Could you check a few things on this model? Use its own coordinates, in mm. A direction names the side the tool comes from. Coordinates: 2 decimals unless noted, no trailing zeros. Order: outer loops, then holes, each group sorted by start corner. A loop starts at its lowest first (then second) coordinate and runs counter-clockwise, first axis right, second up. Notation, with made-up numbers: M 10.25,7 L 41.25,7 A21 cw 41.25,43 Z; hole C 38,30 d11. An arc over 180 degrees is marked long. Put each result on its own line as item: value. Start each with the question number.
```python
from build123d import *

# Parameters (mm, degrees)
EXTRUDE_3_DEPTH     = 13
SKETCH_5_R          = 2.1
CUT_EXTRUDE_2_DEPTH = 48.895720059
SKETCH_6_W          = 7.2
SKETCH_6_H          = 35
EXTRUDE_4_DEPTH     = 20
SKETCH_7_R          = 2.1
CUT_EXTRUDE_3_DEPTH = 20
SKETCH_8_W          = 22.8
SKETCH_8_H          = 3.5
EXTRUDE_5_DEPTH     = 10
SKETCH_9_R          = 6.65
CUT_EXTRUDE_4_DEPTH = 4.2
CUT_EXTRUDE_5_DEPTH = 10
CUT_EXTRUDE_6_DEPTH = 10
SKETCH_14_R         = 6.85
SKETCH_14_R_2       = 5.65
EXTRUDE_7_DEPTH     = 3


with BuildPart() as part:
    # 草图4 → 凸台-拉伸3 (new body)
    with BuildSketch(Plane.XY):
        Polygon((15, 0), (-15, 0), (-15, 35), (-7.8, 35), (-7.8, 3.5), (7.8, 3.5), (7.8, 35), (15, 35), align=None)
    extrude(amount=EXTRUDE_3_DEPTH)

    # 草图5 → 切除-拉伸2 (cut, through all)
    with BuildSketch(Plane(origin=(15, 0, 0), x_dir=(0, 0, -1), z_dir=(1, 0, 0))):
        with Locations(Location((-6.5, 30, 0), (0, 0, 90))):
            Circle(SKETCH_5_R)
    extrude(amount=-CUT_EXTRUDE_2_DEPTH, mode=Mode.SUBTRACT)

    # 草图6 → 凸台-拉伸4 (add)
    with BuildSketch(Plane.XY.offset(13)):
        with Locations((-11.4, 17.5)):
            Rectangle(SKETCH_6_W, SKETCH_6_H)
    extrude(amount=EXTRUDE_4_DEPTH)

    # 草图7 → 切除-拉伸3 (cut)
    with BuildSketch(Plane.ZY.offset(15)):
        with Locations(Location((23.849351573, 12, 0), (0, 0, 270))):
            Circle(SKETCH_7_R)
    extrude(amount=-CUT_EXTRUDE_3_DEPTH, mode=Mode.SUBTRACT)

    # 草图8 → 凸台-拉伸5 (add)
    with BuildSketch(Plane.XY.offset(13)):
        with Locations((3.6, 1.75)):
            Rectangle(SKETCH_8_W, SKETCH_8_H)
    extrude(amount=EXTRUDE_5_DEPTH)

    # 草图9 → 切除-拉伸4 (cut)
    with BuildSketch(Plane(origin=(-7.8, 0, 0), x_dir=(0, 0, -1), z_dir=(1, 0, 0))):
        with Locations(Location((-23.849351573, 12, 0), (0, 0, 90))):
            Circle(SKETCH_9_R)
    extrude(amount=-CUT_EXTRUDE_4_DEPTH, mode=Mode.SUBTRACT)

    # 草图10 → 切除-拉伸5 (cut)
    with BuildSketch(Plane.ZY.offset(15)):
        Polygon((12.890771142, 35), (31.03620252, 14.67169088), (31.03620252, 9.814342957), (24.670130024, 0), (33, 0), (33, 10.134215088), (33, 35), align=None)
        Polygon((0, 35), (0, 31.107929111), (4.419316467, 35), align=None)
    extrude(amount=-CUT_EXTRUDE_5_DEPTH, mode=Mode.SUBTRACT)

    # 草图11 → 切除-拉伸6 (cut)
    with BuildSketch(Plane(origin=(15, 0, 0), x_dir=(0, 0, -1), z_dir=(1, 0, 0))):
        Polygon((-3.336766509, 35), (0, 31.348169844), (0, 35), align=None)
        Polygon((-10.303751585, 35), (-13, 35), (-13, 31.657050955), align=None)
    extrude(amount=-CUT_EXTRUDE_6_DEPTH, mode=Mode.SUBTRACT)

    # 草图14 → 凸台-拉伸7 (add)
    with BuildSketch(Plane.ZY.offset(15)):
        with Locations(Location((23.849351573, 12, 0), (0, 0, 180))):
            Circle(SKETCH_14_R)
        with Locations((23.849351573, 12)):
            Circle(SKETCH_14_R_2, mode=Mode.SUBTRACT)
    extrude(amount=EXTRUDE_7_DEPTH)


solid = part.part
```
Item 1: If we section it at B-B on x = 8.5: Write out the boundary of the cut face in (y, z), then the cut area to 3 significant figures.
Item 2: If we section it at A-A on y = 12: Write out the boundary of the cut face in (x, z), then the cut area to 3 significant figures.
Item 3: If we section it at D-D on y = 30: Write out the boundary of the cut face in (x, z).
Item 4: If we mould it in two halves opening along Z, with no side actions, what happens to faces 1 (the flat face through (0, 0, 12)), 2 (the flat face through (10, 16, 0)), 3 (the flat face through (-12, 10, 25))? For each: released by +Z, released by -Z, zero draft, split by the parting line, or undercut.
Item 5: I need wall thicknesses on probe 1 along X at (y, z) = (5, 2); probe 2 along X at (y, z) = (24, 17); probe 3 along Z at (x, y) = (12, 23). Which ranges of each line are inside material? Lowest first, please.
Item 6: For pin 1 Ø2 at (x, y) = (10, 14.5) entering from +Z; pin 2 Ø6.5 at (y, z) = (12, 23.85) entering from -X; pin 3 Ø3 at (x, y) = (-1, 2) entering from +Z, each with a flat end and sliding along its axis, tell me the tip position at first contact or that it passes through.
Item 7: For faces 4 (the cylindrical face through (-16.48, 7.37, 28.9)), 5 (the flat face through (7.8, 19, 6)), 6 (the flat face through (3, 2, 23)), 7 (the flat face through (-11.45, 33.03, 2.18)), which set-ups out of +Z, -Z, +X, -X, +Y, -Y let a thin tool reach every point of the face, with its end or its side?
Item 8: If we section it at C-C on z = 6.5: Write out the boundary of the cut face in (x, y).
Geometry check:
1. outline: M 0,0 L 31.35,0 L 35,3.34 L 35,10.3 L 31.66,13 L 3.5,13 L 3.5,23 L 0,23 Z; hole C 30,6.5 d4.2
1. area: 466 mm²
2. outline: M -18,17 L -15,17 L -15,0 L -7.8,0 L -7.8,17.2 L -12,17.2 L -12,21.75 L -15,21.75 L -15,18.2 L -18,18.2 Z; M -18,29.5 L -15,29.5 L -15,25.95 L -12,25.95 L -12,30.5 L -7.8,30.5 L -7.8,31.04 L -15,31.04 L -15,30.7 L -18,30.7 Z; M 7.8,0 L 15,0 L 15,13 L 7.8,13 Z
2. area: 256 mm²
3. outline: M -15,0 L -7.8,0 L -7.8,4.4 L -15,4.4 Z; M -15,8.6 L -7.8,8.6 L -7.8,17.35 L -15,17.35 Z; M 7.8,0 L 15,0 L 15,4.4 L 7.8,4.4 Z; M 7.8,8.6 L 15,8.6 L 15,13 L 7.8,13 Z
4. face 1: zero draft
4. face 2: released by -Z
4. face 3: undercut
5. probe 1: x = -15 to -7.8, 7.8 to 15
5. probe 2: x = -15 to -7.8
5. probe 3: z = 0 to 13
6. pin 1: stops at z = 13
6. pin 2: stops at x = -15
6. pin 3: stops at z = 23
7. face 4: -X
7. face 5: +Z, -Z, +Y
7. face 6: +Z, +X, +Y, -Y
7. face 7: -Z, -X, +Y
8. outline: M -15,0 L 15,0 L 15,27.9 L 7.8,27.9 L 7.8,3.5 L -7.8,3.5 L -7.8,27.9 L -15,27.9 Z; M -15,32.1 L -7.8,32.1 L -7.8,35 L -15,35 Z; M 7.8,32.1 L 15,32.1 L 15,35 L 7.8,35 Z
